Geometry: see drawing. Coordinates: mm, zero at the bounding-box minimum. Give positions to 0.01 mm unless a question says otherwise; leave off trailing zeros. Write each loop counter-clockwise with the first axis right and the second up, starting at its lowest first coordinate (ties: lowest second). Pieces come first, ordered by that corner, then holes. Notation, with made-up numbers: (-21, 63) -> (-9, 63) arc R16 cw to (-9, 79) -> close; hole circle Ø9 at (-9.75, 34.5). An arc over 180 degrees is marked (long way). Use CSV: the item, a comma, the result in double quotes. Start each with the question number.
1) Section C-C (z = 9.5). Output: boundary loops of the cut face in (x, y).
2) Section B-B (x = 5.25). Output: boundary loops of the cut face in (y, z), plus the area to 4 significant figures.
3) Section D-D (x = 2.5). Output: boundary loops of the cut face in (y, z).
4) Section A-A (y = 2.45). Output: boundary loops of the cut face in (x, z).
5) Draft query along X for the marked faces 1 and 2. Return one class per face: pulls with the +X half, pulls with the -X half, needs draft (parallel to the pull), parting line crosses it, or undercut.
6) Contact query for flat-ended pins moving along their axis: P1, Ø0.8, axis at y = 2, z = 21, coming from the +X side; P2, Ø0.8, axis at y = 2, z = 20, coming from the -X side; P3, Ø14, axis at x = 12.5, z = 29.5, coming from the +Y side. Output: stop coordinate, or through.
7) Material intervals for line 1 (X direction, y = 1.65, z = 35); line 2 (Z direction, x = 19, y = 2.45); line 3 (Y direction, x = 8.25, z = 13), sorted ascending. Write a range as [from, to].
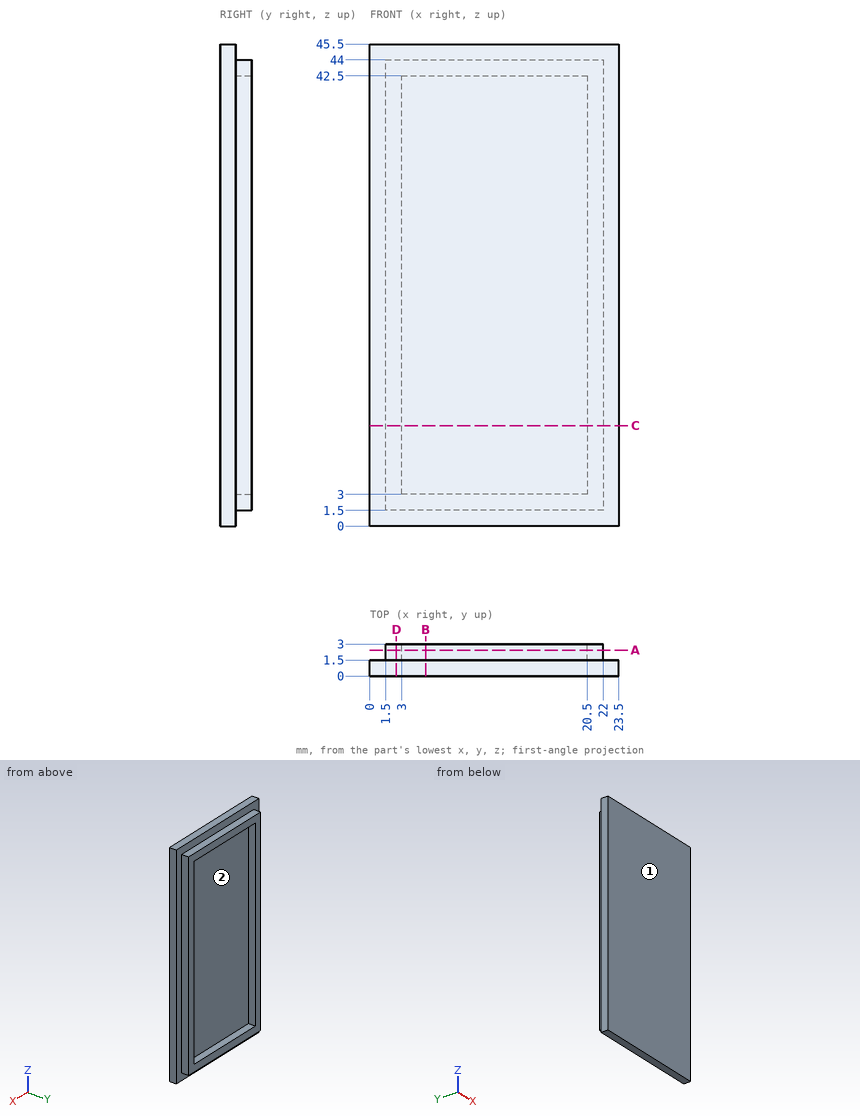
Answers follow:
1,outline,"(0, 0) -> (23.5, 0) -> (23.5, 1.5) -> (22, 1.5) -> (22, 3) -> (20.5, 3) -> (20.5, 1.5) -> (3, 1.5) -> (3, 3) -> (1.5, 3) -> (1.5, 1.5) -> (0, 1.5) -> close"
2,outline,"(0, 0) -> (1.5, 0) -> (1.5, 1.5) -> (3, 1.5) -> (3, 3) -> (1.5, 3) -> (1.5, 42.5) -> (3, 42.5) -> (3, 44) -> (1.5, 44) -> (1.5, 45.5) -> (0, 45.5) -> close"
2,area,"72.75 mm^2"
3,outline,"(0, 0) -> (1.5, 0) -> (1.5, 1.5) -> (3, 1.5) -> (3, 44) -> (1.5, 44) -> (1.5, 45.5) -> (0, 45.5) -> close"
4,outline,"(1.5, 1.5) -> (22, 1.5) -> (22, 44) -> (1.5, 44) -> close; hole (3, 3) -> (20.5, 3) -> (20.5, 42.5) -> (3, 42.5) -> close"
5,face 1,"needs draft"
5,face 2,"undercut"
6,P1,"stops at x = 22"
6,P2,"stops at x = 1.5"
6,P3,"stops at y = 1.5"
7,line 1,"x = [1.5, 3], [20.5, 22]"
7,line 2,"z = [1.5, 3], [42.5, 44]"
7,line 3,"y = [0, 1.5]"
